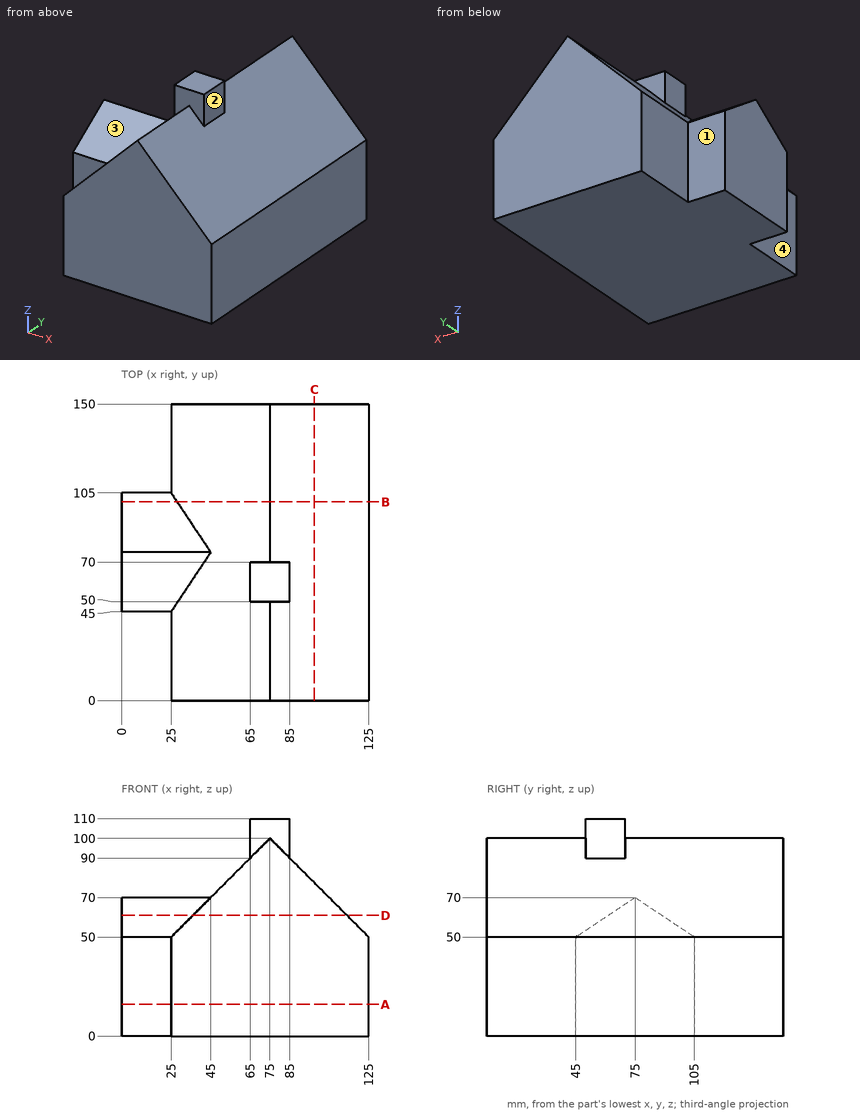
Study the drawing (mm; zero at the part's minimum x, y, z) and answer. A direction names the side the tool comes from. Coordinates: 2 decimals unless noted, no trailing zeros. Order: outer loops, then holes, each group sorted by start corner. A loop starts at its lowest first (then second) coordinate and runs counter-clockwise, first axis right, second up. Notation, with made-up numbers: (-4.75, 77) -> (6.25, 77) arc R22 ccw to (6.25, 102) -> close; hole circle Ø1 at (48, -5.75). An arc over 180 degrees is marked (long way). Answer in a Markdown table with one row per item. Add a question column.
Item 1: Find section D-D (z = 61). Write down the section's boundary in (x, y), then the cut area to 3 significant figures.
Item 2: Find section A-A (z = 16). Write down the section's boundary in (x, y).
Item 3: Each of these flat-tipped pins is pushed along its axis until it touches: P1, Ø5, axis at y = 96.5, z = 90.5, coming from the -X side; P2, Ø12, axis at x = 91.5, y = 85.5, coming from the +Z side; P3, Ø7.5, axis at x = 15, z = 30, coming from the -Y side. Where does it stop, or does it pass through?
Item 4: Find section B-B (y = 100.5). Write down the section's boundary in (x, z).
Item 5: Find the intervals of material crossed by L1, parallel to Y at x = 22.5, z = 50; L2, parallel to Z at x = 50, y = 79; L3, parallel to Z at x = 90, y = 143, in increasing order. Write a range as from..to.
Item 6: Find section C-C (x = 97.5). Write down the section's boundary in (y, z).
Item 7: Which of the six approach directions +Z, -Z, +X, -X, +Y, -Y give full straight-line access (tool end or side, diameter ignored) to the marked faces 1, 2, 3 and 4?
Result set:
| question | item | result |
|---|---|---|
| 1 | outline | (0, 61.5) -> (36, 61.5) -> (36, 0) -> (114, 0) -> (114, 150) -> (36, 150) -> (36, 88.5) -> (0, 88.5) -> close |
| 1 | area | 12,700 mm² |
| 2 | outline | (0, 45) -> (25, 45) -> (25, 0) -> (125, 0) -> (125, 150) -> (25, 150) -> (25, 105) -> (0, 105) -> close |
| 3 | P1 | stops at x = 63 |
| 3 | P2 | stops at z = 89.5 |
| 3 | P3 | stops at y = 45 |
| 4 | outline | (0, 0) -> (125, 0) -> (125, 50) -> (75, 100) -> (28, 53) -> (0, 53) -> close |
| 5 | L1 | y = 45..105 |
| 5 | L2 | z = 0..75 |
| 5 | L3 | z = 0..85 |
| 6 | outline | (0, 0) -> (150, 0) -> (150, 77.5) -> (0, 77.5) -> close |
| 7 | face 1 | +Z, -Z, -X, +Y |
| 7 | face 2 | +Z, +X, +Y, -Y |
| 7 | face 3 | +Z, -X, -Y |
| 7 | face 4 | +Z, -Z, -X, -Y |
